Check sheet for the modelled part. Datum: model origin and axes. Units: mm. A direction names the side the tool comes from. Give positions to 0.01 mm unless a question says otherwise; leave off trailing zeros. Write each loop counter-clockwise with the first axis right and the second up, starting at its lowest first coordinate (ties: lowest second). Pieces come first, ordered by that corner, then holes. Notation, with made-up numbers: (2, 19) - (13, 19) arc R10 cw to (13, 29) - close; hole circle Ø7 at (77, 81). An arc over 180 degrees is marked (long way). Return JSON: item names as keys, results as strings. Group by question number.
```python
from build123d import *

# Parameters (mm, degrees)
F0_W     = 508
F0_H     = 25.4
F0_R     = 6.35
F1_DEPTH = 254


with BuildPart() as f1:
    # F0 (on Front) → F1 (new body, symmetric)
    with BuildSketch(Plane.XZ):
        with Locations((9.227537, 0)):
            Rectangle(F0_W, F0_H)
        with Locations((-190.37859, 0)):
            Circle(F0_R, mode=Mode.SUBTRACT)
        with Locations((190.37859, 0)):
            Circle(F0_R, mode=Mode.SUBTRACT)
    extrude(amount=F1_DEPTH, both=True)

    # F3 (on offset) → F4 (revolve)
    with BuildSketch(Plane.XZ.offset(101.6)):
        with BuildLine():
            ThreePointArc((-101.6, 23.286832), (-109.828136, 25.325427), (-116.152795, 30.969607))
            Line((-116.152795, 30.969607), (-116.152795, 10.770973))
            Line((-116.152795, 10.770973), (-101.6, 10.770973))
            Line((-101.6, 10.770973), (-101.6, 23.286832))
        make_face()
    revolve(axis=Axis((-101.6, -101.6, 17.028903), (0, 0, -1)))

    # F5: F1 across plane


with BuildPart() as f1_1:
    add(f1.part)
    add(f1.part.mirror(Plane.YZ))

    # F6: F1 across plane


with BuildPart() as f1_2:
    add(f1_1.part)
    add(f1_1.part.mirror(Plane.XZ))


solid = f1_2.part
```
Item 1: Section check A-A on z = 0. Record the cut outline in (x, y).
Item 2: Mould release check, pull along Y, two halves, no side actions. Record for faces 1 (the face through (-109.423, -89.329, 21.707)), 2 (the face through (263.228, -4, 0)), 3 (the face through (-4, 254, 0)), 4 (the face through (-4, -254, 0)): +Y half, -Y half, draft (parallel to the pull), parting line (faces both ways), or undercut.
Item 3: Depth check by flat-ended pin: pin 1 (2 mm diameter, centred on y = 98, z = 24, fed in from -X); pin 2 (7.5 mm diameter, centred on x = 190.38, z = 0, fed in from -Y). Enter the tip coordinate at first touch or a pass-through.
Item 4: Material ranges on line 1 along X through (y, z) = (-57.5, 0); line 2 along X through (y, z) = (150, -1); line 3 along Z through (x, y) = (55.5, -64.5), recorded low to high. Write a range as from..to.
Item 5: Section check B-B on y = -148. Record the cut outline in (x, z), plus the area to 3 significant figures.
Item 6: Section check C-C on x = -60. Record the cut outline in (y, z), plus the area to 3 significant figures.
Item 7: Access from +Z, -Z, +X, -X, +Y, -Y to the whole of each face (thin tool, end or side, straight path). Record for faces 5 (the face through (-4, -4, -12.7)), 6 (the face through (109.423, 89.329, 21.707)).
Reply:
{
 "1": {"outline": "(-263.23, -254) - (-196.73, -254) - (-196.73, 254) - (-263.23, 254) - close; (-184.03, -254) - (184.03, -254) - (184.03, 254) - (-184.03, 254) - close; (196.73, -254) - (263.23, -254) - (263.23, 254) - (196.73, 254) - close"},
 "2": {"face 1": "undercut", "face 2": "draft", "face 3": "+Y half", "face 4": "-Y half"},
 "3": {"pin 1": "x = -115.92", "pin 2": "through"},
 "4": {"line 1": "-263.23..-196.73, -184.03..184.03, 196.73..263.23", "line 2": "-263.23..-196.65, -184.11..184.11, 196.65..263.23", "line 3": "-12.7..12.7"},
 "5": {"outline": "(-263.23, -12.7) - (263.23, -12.7) - (263.23, 12.7) - (-263.23, 12.7) - close; hole circle Ø12.7 at (-190.38, 0); hole circle Ø12.7 at (190.38, 0)", "area": "13,100 mm²"},
 "6": {"outline": "(-254, -12.7) - (254, -12.7) - (254, 12.7) - (-254, 12.7) - close", "area": "12,900 mm²"},
 "7": {"face 5": "-Z, +X, -X, +Y, -Y", "face 6": "+Z"}
}
